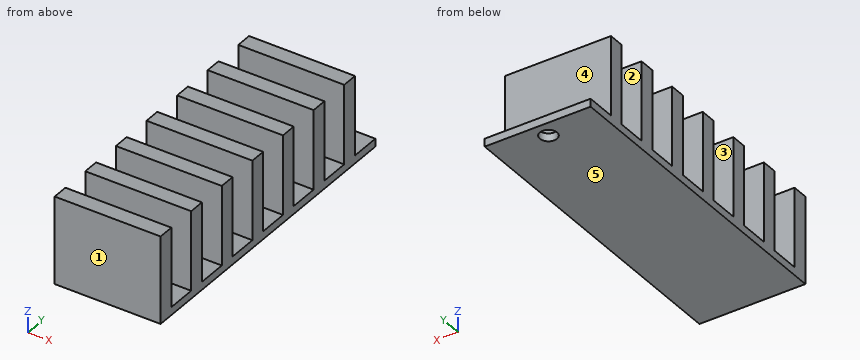
from build123d import *

# Parameters (mm, degrees)
F0_W     = 50.8
F0_H     = 152.4
F1_DEPTH = 3.81
F2_W     = 50.8
F2_H     = 7.62
F3_DEPTH = 38.1
F4_R     = 4.120653
F5_DEPTH = 25.4


with BuildPart() as f1:
    # F0 (on Top) → F1 (new body)
    with BuildSketch(Plane.XY):
        with Locations((25.4, 76.2)):
            Rectangle(F0_W, F0_H)
    extrude(amount=F1_DEPTH)

    # F2 (on face) → F3 (join)
    with BuildSketch(Plane.XY.offset(3.81)):
        with Locations((25.4, 134.13)):
            Rectangle(F2_W, F2_H)
        with Locations((25.4, 112.41)):
            Rectangle(F2_W, F2_H)
        with Locations((25.4, 90.69)):
            Rectangle(F2_W, F2_H)
        with Locations((25.4, 68.97)):
            Rectangle(F2_W, F2_H)
        with Locations((25.4, 47.25)):
            Rectangle(F2_W, F2_H)
        with Locations((25.4, 3.81)):
            Rectangle(F2_W, F2_H)
        with Locations((25.4, 25.53)):
            Rectangle(F2_W, F2_H)
    extrude(amount=F3_DEPTH)

    # F4 (on face) → F5 (cut)
    with BuildSketch(Plane.XY.offset(3.81)):
        with Locations((25.4, 144.709066)):
            Circle(F4_R)
    extrude(amount=-F5_DEPTH, mode=Mode.SUBTRACT)


solid = f1.part
Verification items for the finished model (mm, model axes). Face numbers are marked on the shaded views. A direction names the side the tool comes from. Round coordinates to 2 decimals unless told otherwise and drop trailing zeros. Write each loop counter-clockwise with the first axis right and the second up, starting at its lowest first coordinate (ties: lowest second). Pieces come first, ordered by that corner, then holes.
(1) Access from +Z, -Z, +X, -X, +Y, -Y to the whole of each face (thin tool, end or side, straight path). Record for the marked faces 1 and 2.
Returned:
face 1: +Z, -Z, +X, -X, -Y
face 2: +Z, +X, -X
(2) Depth check by flat-ended pin: pin 1 Ø11.5 at (x, z) = (21.5, 19.5) entering from +Y; pin 2 Ø8 at (y, z) = (102, 28.5) entering from +X; pin 3 Ø11.5 at (x, y) = (21.5, 148.5) entering from +Z. Enter the tip coordinate at first touch or a pass-through.
Returned:
pin 1: stops at y = 137.94
pin 2: passes through
pin 3: stops at z = 3.81
(3) Section check B-B (z = 25.5). Enter the section's corners in (x, y).
Returned:
outline: (0, 0) - (50.8, 0) - (50.8, 7.62) - (0, 7.62) - close; (0, 21.72) - (50.8, 21.72) - (50.8, 29.34) - (0, 29.34) - close; (0, 43.44) - (50.8, 43.44) - (50.8, 51.06) - (0, 51.06) - close; (0, 65.16) - (50.8, 65.16) - (50.8, 72.78) - (0, 72.78) - close; (0, 86.88) - (50.8, 86.88) - (50.8, 94.5) - (0, 94.5) - close; (0, 108.6) - (50.8, 108.6) - (50.8, 116.22) - (0, 116.22) - close; (0, 130.32) - (50.8, 130.32) - (50.8, 137.94) - (0, 137.94) - close
(4) Mould release check, pull along Y, two halves, no side actions. Record for the marked faces 3, 4 and 5: pulls with the +Y half, pulls with the -Y half, needs draft (parallel to the pull), parting line crosses it, or undercut.
Returned:
face 3: undercut
face 4: pulls with the +Y half
face 5: needs draft
(5) Material ranges on line 1 (Y direction, x = 25.4, z = 2.95); line 2 (Z direction, x = 19.5, y = 84), recorded low to high.
Returned:
line 1: y = 0 to 140.59, 148.83 to 152.4
line 2: z = 0 to 3.81
(6) Section check D-D (y = 37). Enter the section's corners in (x, z).
Returned:
outline: (0, 0) - (50.8, 0) - (50.8, 3.81) - (0, 3.81) - close
